Model file for the job. Use its own axes, mm. A direction names the side the tool comes from. Give positions to 0.01 mm unless a question says otherwise; leave off trailing zeros. Loops run counter-clockwise (first coordinate to the right, second up) from the corner with the lowest first, then second, coordinate; pieces in that order, holes last. Notation, with made-up numbers: (9.25, -38.5) -> (66.25, -38.5) arc R28 cw to (66.25, -7.5) -> close; hole circle Ø4 at (-23, 59). An arc over 180 degrees is marked (long way). Use CSV: the item, a comma, the result in double quotes. Start each with the question number.
(1) Pull direction Y, two halves, no side cores. Call faces 1 (the cylindrical face through (-4.764, -34.923, -0.07)), 2 (the flat face through (-32.824, -28.954, 0.071)), 3 (the flat face through (-9, -39.243, 0)), 4 (the flat face through (-33.22, -1.65, 0.07)): pulls with the +Y half, pulls with the -Y half, needs draft (parallel to the pull), parting line crosses it, or undercut.
(2) Drill centre lines: probe 1 along X at (y, z) = (-25.6, 0); probe 2 along Z at (x, y) = (-6.5, -36); probe 3 along Y at (x, z) = (-10, 2.5). Where is each one in solid material? Low to high.
(3) Cut at A-A on x = -54. Write the cut outline in (y, z).
(4) Flat gauge pins, fed straight in: pin 1 (4 mm diameter, centred on x = -47, z = 0.5, fed in from -Y); pin 2 (3.5 mm diameter, centred on x = -57.15, z = 0, fed in from -Y); pin 3 (3 mm diameter, centred on y = -11, z = 2, fed in from +X). Where does each tip first touch, or does it go through?
(5) Cut at B-B on y = -3.5. State how many separate pieces and enclosed holes the cut face has, then the cut area to 3 significant figures.
(6) Cut at C-C on y = -17.5. Write the cut outline in (x, z), then the cut area to 3 significant figures.
(7) 3-axis set-ups, long thin cutter, end or side, ignore diameter. For faces 5 (the flat face through (-46, 3.81, -2)), 6 (the flat face through (-9, 0, 0)), 7 (the cylindrical face through (-45.29, -31.2, 0.71)): which of +Z, -Z, +X, -X, +Y, -Y reach the whole face in a straight line?
Autodesk Inventor part; units mm, degrees
ref_plane "YZ Plane" through (0, 0, 0) normal (1, 0, 0) x (0, 1, 0)
ref_plane "XZ Plane" through (0, 0, 0) normal (0, 1, 0) x (-1, 0, 0)
ref_plane "XY Plane" through (0, 0, 0) normal (0, 0, 1) x (1, 0, 0)
ref_plane "Work Plane1" through (0, -15.24, 5.08) normal (0, 1, 0) x (-1, 0, 0)
sketch "Sketch2" plane through (0, -15.24, 0) normal (0, 1, 0) x (-1, 0, 0)
  arc A0 (6.35, -5.08) -> (6.35, 5.08) centre (6.35, 0) ccw construction
  line L0 (6.35, 5.08) -> (0, 5.08)
  line L1 (0, -5.08) -> (6.35, -5.08)
  circle A1 centre (6.35, 0) radius 1.5875
  arc A2 (6.35, 5.08) -> (6.35, -5.08) centre (6.35, 0) ccw
  line L2 (6.35, 5.08) -> (57.15, 5.08)
  line L3 (6.35, -5.08) -> (57.15, -5.08)
  arc A3 (57.15, -5.08) -> (57.15, 5.08) centre (57.15, 0) ccw
  arc A4 (6.35, -5.08) -> (6.35, 5.08) centre (6.35, 0) ccw construction
  arc A5 (57.15, 5.08) -> (57.15, -5.08) centre (57.15, 0) ccw construction
  point P0 (0, 0)
  dimension "d0" = 50.8
extrude "Extrusion1" add sketch "Sketch2" along normal mid plane 48.006
sketch "Sketch3" plane through (-57.15, 8.763, 5.08) normal (0, 0, 1) x (1, 0, 0)
  line L0 (57.15, -8.763) -> (57.15, -39.243)
  line L1 (50.8, -8.763) -> (57.15, -8.763)
  line L2 (50.8, -8.763) -> (50.8, -39.243)
  line L3 (57.15, -39.243) -> (50.8, -39.243)
  line L4 (55.88, -48.006) -> (55.88, 0)
  line L5 (55.88, -39.243) -> (55.88, -8.763)
  line L6 (55.88, -8.763) -> (43.18, -8.763)
  line L7 (43.18, -8.763) -> (43.18, -39.243)
  line L8 (5.08, -11.049) -> (40.005, 0)
  line L9 (50.8, 0) -> (0, 0)
  line L10 (0, -48.006) -> (0, 0) construction
  line L11 (0, 0) -> (0, 0)
  line L12 (0, -48.006) -> (0, 0) construction
  line L13 (0, -48.006) -> (0, -48.006)
  line L14 (40.005, 0) -> (55.88, 0) construction
  line L15 (55.88, -24.003) -> (-5.08, -24.003) construction
  line L16 (40.005, 0) -> (-5.08, 0)
  line L17 (-5.08, -11.049) -> (-5.08, 0)
  line L18 (5.08, -36.957) -> (40.005, -48.006)
  line L19 (5.08, -36.957) -> (-5.08, -36.957)
  line L20 (40.005, -48.006) -> (55.88, -48.006) construction
  line L21 (50.8, -48.006) -> (0, -48.006)
  line L22 (-5.08, -48.006) -> (0, -48.006)
  line L23 (-5.08, -48.006) -> (-5.08, 0) construction
  line L24 (40.005, -48.006) -> (-5.08, -48.006)
  line L25 (-5.08, -36.957) -> (-5.08, -48.006)
  line L26 (0, -48.006) -> (0, 0) construction
  line L27 (5.08, -11.049) -> (-5.08, -11.049)
  line L28 (5.08, -36.957) -> (5.08, -11.049) construction
  line L29 (55.88, -39.243) -> (43.18, -39.243)
  dimension "d3" = 15.875
  dimension "d5" = 25.908
  dimension "d10" = 10.16
  dimension "d17" = 12.7
extrude "Extrusion2" cut sketch "Sketch3" against normal through all
sketch "Sketch4" plane through (-57.15, -2.286, 0) normal (0, 1, 0) x (1, 0, 0)
  arc A0 (0, 5.08) -> (0, -5.08) centre (0, 0) ccw
  circle A1 centre (0, 0) radius 1.5875
  circle A2 centre (50.8, 0) radius 1.5875
  point P0 (57.15, 0)
extrude "Extrusion3" cut sketch "Sketch4" against normal through all contours A1
sketch "Sketch6" plane through (-17.145, -39.243, 5.08) normal (0, 0, 1) x (1, 0, 0)
  line L0 (-45.085, 11.049) -> (-45.085, 36.957)
  line L1 (-40.005, 11.049) -> (-45.085, 11.049)
  line L2 (-40.005, 11.049) -> (-34.925, 11.049)
  line L3 (-45.085, 36.957) -> (-40.005, 36.957)
  line L4 (-34.925, 36.957) -> (-40.005, 36.957)
  line L5 (-45.085, 31.623) -> (-34.925, 31.623)
  line L6 (-34.925, 31.623) -> (-34.925, 16.383)
  line L7 (-34.925, 16.383) -> (-45.085, 16.383)
  line L8 (-45.085, 16.383) -> (-45.085, 31.623)
  line L9 (-45.085, 31.623) -> (-34.925, 16.383) construction
  line L10 (-34.925, 31.623) -> (-45.085, 16.383) construction
  line L11 (-40.005, 24.003) -> (-45.085, 24.003) construction
  point P0 (17.145, 39.243)
  dimension "d19" = 10.16
  dimension "d20" = 15.24
extrude "Extrusion5" cut sketch "Sketch6" against normal through all
sketch "Sketch5" plane through (-17.145, -39.243, 5.08) normal (0, 0, 1) x (1, 0, 0)
  line L0 (-40.005, 11.049) -> (-34.925, 11.049)
  line L1 (-34.925, 11.049) -> (0, 0)
  line L2 (10.795, 0) -> (0, 0)
  line L3 (10.795, 0) -> (10.795, 8.763)
  line L4 (10.795, 39.243) -> (10.795, 48.006)
  line L5 (0, 48.006) -> (10.795, 48.006)
  line L6 (0, 48.006) -> (-34.925, 36.957)
  line L7 (-34.925, 36.957) -> (-40.005, 36.957)
  line L8 (-40.005, 11.049) -> (-40.005, 16.383)
  line L9 (10.795, 8.763) -> (3.175, 8.763)
  line L10 (3.175, 8.763) -> (3.175, 39.243)
  line L11 (3.175, 39.243) -> (10.795, 39.243)
  line L12 (-40.005, 31.623) -> (-34.925, 31.623)
  line L13 (-34.925, 31.623) -> (-34.925, 16.383)
  line L14 (-34.925, 16.383) -> (-40.005, 16.383)
  line L15 (-40.005, 31.623) -> (-40.005, 36.957)
  line L16 (-1.905, 5.9308) -> (-29.845, 14.77)
  line L17 (-29.845, 14.77) -> (-29.845, 33.236)
  line L18 (-29.845, 33.236) -> (-1.905, 42.0752)
  line L19 (-1.905, 42.0752) -> (-1.905, 5.9308)
  dimension "d23" = 5.08
extrude "Extrusion4" cut sketch "Sketch5" against normal through all contours L16 L17 L18 L19
sketch "Sketch8" plane through (0, -15.24, 5.08) normal (0, 1, 0) x (-1, 0, 0)
  circle A0 centre (46.99, -5.08) radius 3.81
  arc A1 (57.15, -10.16) -> (57.15, 0) centre (57.15, -5.08) ccw
  line L0 (62.23, -5.08) -> (46.99, -5.08) construction
  point P0 (0, -5.08)
  dimension "d24" = 7.62
  dimension "d25" = 15.24
extrude "Extrusion6" add sketch "Sketch8" along normal mid plane 38.1
sketch "Sketch9" plane through (-46.99, 3.81, 0) normal (0, 1, 0) x (1, 0, 0)
  circle A0 centre (0, 0) radius 1.8415
  circle A1 centre (0, 0) radius 3.81
  point P0 (46.99, 0)
  dimension "d28" = 3.683
extrude "Extrusion7" cut sketch "Sketch9" against normal through all contours A0
ref_plane "Work Plane2" through (-46.99, 16.51, 0) normal (0, 1, 0) x (1, 0, 0)
sketch "Sketch10" plane through (-46.99, 16.51, 0) normal (0, 1, 0) x (1, 0, 0)
  circle A0 centre (0, 0) radius 1.8415
  circle A1 centre (0, 0) radius 1.8415
  point P0 (46.99, 0)
extrude "Extrusion8" add sketch "Sketch10" against normal up to surface (44.704 mm away)
sketch "Sketch11" plane through (-46.99, 16.51, 0) normal (0, 1, 0) x (1, 0, 0)
  circle A0 centre (0, 0) radius 3.81
  circle A1 centre (0, 0) radius 3.4925
  point P0 (46.99, 0)
  dimension "d34" = 6.985
extrude "Extrusion9" add sketch "Sketch11" along normal blind 2.54 contours A1
full round fillet "Fillet1" first side at (-44.0995, 16.51, 0.4255) centre faces at (-43.5088, 18.2033, 0.281) second side at (-46.6012, 19.05, -0.8909)
properties part number "A_Arm"
Check result:
1,face 1,"needs draft"
1,face 2,"undercut"
1,face 3,"pulls with the -Y half"
1,face 4,"undercut"
2,probe 1,"-62.23 to -58.74, -55.56 to -43.18, -19.05 to -13.97"
2,probe 2,"-5.08 to -1.58, 1.58 to 5.08"
2,probe 3,"-39.24 to -30.48, 0 to 8.76"
3,outline,"(-28.19, -5.08) -> (-22.86, -5.08) -> (-22.86, 5.08) -> (-28.19, 5.08) -> close; (-7.62, -5.08) -> (-2.29, -5.08) -> (-2.29, 5.08) -> (-7.62, 5.08) -> close"
4,pin 1,"y = -34.29"
4,pin 2,"y = -28.19"
4,pin 3,"x = -13.97"
5,separate pieces,"2"
5,enclosed holes,"1"
5,area,"268 mm²"
6,outline,"(-52.07, -5.08) -> (-46.99, -5.08) -> (-46.99, -3.81) arc R3.81 ccw to (-46.99, 3.81) -> (-46.99, 5.08) -> (-52.07, 5.08) -> close; (-19.05, -5.08) -> (-13.97, -5.08) -> (-13.97, 5.08) -> (-19.05, 5.08) -> close"
6,area,"126 mm²"
7,face 5,"none"
7,face 6,"+Z, -Z, +X"
7,face 7,"-Y"
